Read the model definition and answer for the solid it produces. Units are mm, in the model's axes. A direction names the side the tool comes from. Coordinates: 2 decimals unless noted, no trailing zeros. Write each loop counter-clockwise with the first axis right and the second up, starting at its lowest first coordinate (ties: lowest second). Pieces come first, ordered by that corner, then holes. Notation, with made-up numbers: (-4.75, 75.5) -> (12.25, 75.5) arc R19 cw to (12.25, 99.5) -> close; hole circle Ø11 at (-15, 85). An arc over 180 degrees is marked (long way). Use CSV: the item, a comma, the result in double quotes.
Solid Edge part; units mm, degrees
sketch "Sketch1" plane through (0, 0, 0) normal (0, 0, 1) x (1, 0, 0)
  line L0 (-41, -16) -> (41, -16)
  line L1 (41, -16) -> (41, 16)
  line L2 (41, 16) -> (-41, 16)
  line L3 (-41, 16) -> (-41, -16)
  dimension "D1" = 41
  dimension "D2" = 41
extrude "Protrusion1" add sketch "Sketch1" along normal mid plane 12
sketch "Sketch2" plane through (0, 0, 6) normal (0, 0, 1) x (1, 0, 0)
  line L0 (20.5, 16) -> (36.5, 16)
  line L1 (36.5, 16) -> (36.5, -11.5)
  line L2 (36.5, -11.5) -> (12.5, -11.5)
  line L3 (12.5, -11.5) -> (12.5, 12)
  line L4 (12.5, 12) -> (20.5, 12)
  line L5 (20.5, 12) -> (20.5, 16)
  dimension "D1" = 36.5
  dimension "D2" = 20.5
  dimension "D3" = 20.5
  dimension "D4" = 36.5
extrude "v_1_servo_cutout" cut sketch "Sketch2" against normal blind 10
sketch "Sketch3" plane through (0, 0, 6) normal (0, 0, 1) x (0, 1, 0)
  line L0 (-9.5, -36.5) -> (-9.5, -41)
  line L1 (-9.5, -41) -> (-1.5, -41)
  line L2 (-1.5, -41) -> (-1.5, -36.5)
  line L3 (-1.5, -36.5) -> (-9.5, -36.5)
  dimension "D1" = 1.5
extrude "Cutout1" cut sketch "Sketch3" against normal up to vertex (10 mm away)
sketch "Sketch4" plane through (0, 0, 6) normal (0, 0, 1) x (0, 1, 0)
  line L0 (-5, -7.5) -> (5, -7.5)
  line L1 (5, -7.5) -> (5, 7.5)
  line L2 (5, 7.5) -> (-5, 7.5)
  line L3 (-5, 7.5) -> (-5, -7.5)
  dimension "D1" = 5
  dimension "D2" = 5
extrude "Cutout2" cut sketch "Sketch4" against normal up to next
sketch "Sketch5" plane through (0, 16, 0) normal (0, 1, 0) x (1, 0, 0)
  arc A0 (37.5498, 6) -> (40.247, -6) centre (30, -2) cw
  dimension "D1" = 30
extrude "Cutout3" cut sketch "Sketch5" against normal through all material side at (40.781, 16, -0.4232)
mirror "Mirror1" about plane through (0, 0, 0) normal (1, 0, 0) of "v_1_servo_cutout", "Cutout1", "Cutout3"
hole "Hole1" at (30, -16, 2) direction (0, 1, 0) diameter 3.7 depth 30 tip angle 118 start chamfer 0.6 start chamfer angle 45 end chamfer 0.6 end chamfer angle 45
hole "Hole2" at (-30, -16, 2) direction (0, 1, 0) diameter 3.7 depth 30 tip angle 118 start chamfer 0.6 start chamfer angle 45 end chamfer 0.6 end chamfer angle 45
hole "Hole3" at (0, 10, 6) direction (0, 0, -1) diameter 2.75 depth 30 tip angle 118 start chamfer 0.6 start chamfer angle 45 end chamfer 0.6 end chamfer angle 45
hole "Hole4" at (0, -10, 6) direction (0, 0, -1) diameter 2.75 depth 30 tip angle 118 start chamfer 0.6 start chamfer angle 45 end chamfer 0.6 end chamfer angle 45
properties material "Polypropylene, general purpose"
1. A cutting plane is placed at A-A (y = -4). Give the vertices of the cut face in (x, z), and give its area (3 significant figures).
Solutions:
outline,"(-39.22, -4) arc R11 ccw to (-37.55, -6) -> (-7.5, -6) -> (-7.5, 6) -> (-12.5, 6) -> (-12.5, -4) -> close; (7.5, -6) -> (37.55, -6) arc R11 ccw to (39.22, -4) -> (12.5, -4) -> (12.5, 6) -> (7.5, 6) -> close"
area,"224 mm^2"
2. For a pull along Y with two mould halves and no side action, classify faces 1 (the flat face through (-1, 7, -6)), 2 (the flat face through (39, -9.5, 1)), 3 (the flat face through (-1, -16, 0)), 4 (the flat face through (1, 16, 0)) as pulls with the +Y half, pulls with the -Y half, needs draft (parallel to the pull), parting line crosses it, or undercut.
Solutions:
face 1,"needs draft"
face 2,"undercut"
face 3,"pulls with the -Y half"
face 4,"pulls with the +Y half"
3. Find the intervals of material crossed by line 1 along X through (y, z) = (10, -2) (3 decimals); line 2 along Y through (x, z) = (0, 1.25) (3 decimals); line 3 along Y through (x, z) = (19.5, -1.75), in increasing order.
Solutions:
line 1,"x = -40.247 to -36.5, -12.5 to -1.375, 1.375 to 12.5, 36.5 to 40.247"
line 2,"y = -16 to -11.375, -8.625 to -5, 5 to 8.625, 11.375 to 16"
line 3,"y = -16 to -11.5, 12 to 16"
4. A cutting plane is placed at B-B (z = -3.25). Give the number of separate pieces and of enclosed holes in the cut face, and give its area (3 significant figures).
Solutions:
separate pieces,"3"
enclosed holes,"3"
area,"1,070 mm^2"
5. Each of these flat-tipped pins is pushed along its axis until it touches: pin 1 Ø3.5 at (x, z) = (30, 2) entering from -Y; pin 2 Ø5 at (x, z) = (-28, 1) entering from +Y; pin 3 Ø8 at (x, y) = (-21, 1) entering from +Z; pin 4 Ø2 at (y, z) = (13.5, 3.5) entering from -X. Where does it stop, or does it pass through?
Solutions:
pin 1,"passes through"
pin 2,"stops at y = -11.5"
pin 3,"stops at z = -4"
pin 4,"stops at x = -40.99"
6. A tool of negligible diameter and unlimited length cuts with its end or side. For faces 5 (the cylindrical face through (-40.712, 0.224, -0.501)), 6 (the flat face through (-24, -11.5, 1)), 7 (the flat face through (7.5, 0, 0)), from which of +Z, -Z, +X, -X, +Y, -Y can it reach the whole face along a straight path? Write none if from no direction.
Solutions:
face 5,"-X, +Y, -Y"
face 6,"+Z"
face 7,"+Z, -Z"
7. A cutting plane is placed at C-C (x = -30). Give the vertices of the cut face in (y, z), and give its area (3 significant figures).
Solutions:
outline,"(-16, -6) -> (16, -6) -> (16, -4) -> (-11.5, -4) -> (-11.5, -0.45) -> (-12.1, 0.15) -> (-15.4, 0.15) -> (-16, -0.45) -> close; (-16, 4.45) -> (-15.4, 3.85) -> (-12.1, 3.85) -> (-11.5, 4.45) -> (-11.5, 6) -> (-16, 6) -> close"
area,"91.6 mm^2"
